Work out the finished part from the listing and answer in its coordinate system (mm). Give positions to 0.01 mm unless a question says otherwise; leave off trailing zeros. Loops run counter-clockwise (first coordinate to the right, second up) from the corner with the lowest first, then second, coordinate; pieces in that order, holes last. Notation, with made-up numbers: (58, -33.75) - (67, -33.75) arc R22 ccw to (67, -6.75) - close; hole circle Ø5 at (32, -4). An arc over 180 degrees is marked (long way). One line per question, with ' | ' between items. Start each with the question number.
1. Section A-A (z = 1.2) is taken. Give the number of separate pieces and of enclosed holes in the cut face, plus the area to 3 significant figures.
2. Section C-C (x = -40) is taken. Determine the outline of the cut face in (y, z).
3. Section B-B (y = 64.5) is taken. Determine the outline of the cut face in (x, z).
4. Find the intervals of material crossed by line 1 (X direction, y = 100, z = 1.4); line 2 (Y direction, x = 15.5, z = 1.1); line 3 (Y direction, x = 2, z = 2.5), in increasing order.
5. Each of these flat-tipped pins is pushed along its axis until it touches: pin 1 (1 mm diameter, centred on y = 129.5, z = 3, fed in from +X); pin 2 (1.2 mm diameter, centred on y = 173, z = 3, fed in from +X); pin 3 (1.2 mm diameter, centred on x = 12, z = 2.5, fed in from -Y). Where does it stop, or does it pass through?
6. For a pull along X with two mould halves and no side action, classify faces 1 (the face through (34, 195, 2)), 2 (the face through (4, 87, 0)), 3 (the face through (-1.42, 10.78, 1.97)), 4 (the face through (-65.414, -18.312, 1.972)) as released by +X, released by -X, zero draft, split by the parting line, or undercut.
from build123d import *

# Parameters (mm, degrees)
SKETCH_1_R          = 1.5
SKETCH_1_R_2        = 10.875
EXTRUDE_1_DEPTH     = 4
FILLET_3_R          = 15
FILLET_4_R          = 5
FILLET_5_R          = 1
SKETCH_2_W          = 12.5
SKETCH_2_H          = 4
SKETCH_2_R          = 1.4
EXTRUDE_2_DEPTH     = 4
FILLET_6_R          = 5
SKETCH_4_R          = 1.5
SKETCH_4_W          = 11.25
SKETCH_4_H          = 4
CUT_EXTRUDE_2_DEPTH = 227.329405955
CHAMFER_1_SIZE      = 10
FILLET_7_R          = 10
SKETCH_3_R          = 1.5
CUT_EXTRUDE_1_DEPTH = 227.329405955


with BuildPart() as part:
    # Эскиз1 → Бобышка-Вытянуть1 (new body)
    with BuildSketch(Plane.XY):
        Polygon((-100, -14.71), (-30, -22), (30, -22), (30, 171), (55, 171), (55, 176.625), (67.5, 176.625), (67.5, 183.375), (55, 183.375), (55, 189), (30, 189), (30, 203), (-30, 203), (-30, 12.58), (-100, 5.29), (-100, -3.31), (-82.5, -3.31), (-82.5, -6.11), (-100, -6.11), align=None)
        with Locations((-15.5, -15.5)):
            Circle(SKETCH_1_R, mode=Mode.SUBTRACT)
        Circle(SKETCH_1_R_2, mode=Mode.SUBTRACT)
        with Locations((15.5, -15.5)):
            Circle(SKETCH_1_R, mode=Mode.SUBTRACT)
        with Locations((-15.5, 15.5)):
            Circle(SKETCH_1_R, mode=Mode.SUBTRACT)
        with Locations((15.5, 15.5)):
            Circle(SKETCH_1_R, mode=Mode.SUBTRACT)
        with Locations((-22.25, 100)):
            Circle(SKETCH_1_R, mode=Mode.SUBTRACT)
        with Locations((2.55, 100)):
            Circle(SKETCH_1_R, mode=Mode.SUBTRACT)
    extrude(amount=EXTRUDE_1_DEPTH)

    # Скругление3
    fillet_3_edges = [part.edges().sort_by_distance(p)[0] for p in [
        (-30, 12.58, 2),
    ]]
    fillet(fillet_3_edges, radius=FILLET_3_R)

    # Скругление4
    fillet_4_edges = [part.edges().sort_by_distance(p)[0] for p in [
        (-100, -14.71, 2),
        (-100, 5.29, 2),
    ]]
    fillet(fillet_4_edges, radius=FILLET_4_R)

    # Скругление5
    fillet_5_edges = [part.edges().sort_by_distance(p)[0] for p in [
        (-100, -6.11, 2),
        (-100, -3.31, 2),
    ]]
    fillet(fillet_5_edges, radius=FILLET_5_R)

    # Эскиз2 → Бобышка-Вытянуть2 (add, through all)
    # profile 1 of 3: a face of its own
    with BuildSketch(Plane.XY.offset(4)):
        with Locations((-23.75, -24)):
            Rectangle(SKETCH_2_W, SKETCH_2_H)
        with Locations((-23.75, -23.75)):
            Circle(SKETCH_2_R, mode=Mode.SUBTRACT)
    # profile 2 of 3: a face of its own
    with BuildSketch(Plane.XY.offset(4)):
        with Locations((0, -24)):
            Rectangle(SKETCH_2_W, SKETCH_2_H)
    # profile 3 of 3: a face of its own
    with BuildSketch(Plane.XY.offset(4)):
        with Locations((23.75, -24)):
            Rectangle(SKETCH_2_W, SKETCH_2_H)
        with Locations((23.75, -23.75)):
            Circle(SKETCH_2_R, mode=Mode.SUBTRACT)
    extrude(amount=-EXTRUDE_2_DEPTH)

    # Скругление6
    # the kernel refuses this fillet: 5 mm, written as the material it adds along each edge
    with BuildSketch(Plane(origin=(-30, -22, 0), x_dir=(0, -1, 0), z_dir=(0, 0, 1))) as fillet_6_piece_1:
        with BuildLine():
            CenterArc((4.509032444, -4.974021107), FILLET_6_R, 95.843205651, 78.21128084)
            Line((-0.4640718, -4.456107822), (-0.563533885, -4.445749556))
            Line((-0.563533885, -4.445749556), (-0.099462085, 0.010358266))
            Line((-0.099462085, 0.010358266), (0, 0.1))
            ThreePointArc((0, 0.1), (2, 0.1), (3.989819351, 0.099480422))
            Line((3.989819351, 0.099480422), (4, 0))
        make_face()
    extrude(amount=4)

    # Эскиз4 → Вырез-Вытянуть2 (cut, through all)
    with BuildSketch(Plane.XY.offset(4)):
        with Locations((23.75, 180)):
            Circle(SKETCH_4_R)
        with Locations((-23.75, 180)):
            Circle(SKETCH_4_R)
        with Locations((-11.875, 180)):
            Rectangle(SKETCH_4_W, SKETCH_4_H)
        with Locations((11.875, 180)):
            Rectangle(SKETCH_4_W, SKETCH_4_H)
        with Locations((35.625, 180)):
            Rectangle(SKETCH_4_W, SKETCH_4_H)
        with Locations((47.5, 180)):
            Circle(SKETCH_4_R)
    extrude(amount=-CUT_EXTRUDE_2_DEPTH, mode=Mode.SUBTRACT)

    # Фаска1
    chamfer_1_edges = [part.edges().sort_by_distance(p)[0] for p in [
        (30, 171, 2),
        (30, 189, 2),
    ]]
    chamfer(chamfer_1_edges, length=CHAMFER_1_SIZE)

    # Скругление7
    fillet_7_edges = [part.edges().sort_by_distance(p)[0] for p in [
        (40, 171, 2),
        (40, 189, 2),
    ]]
    fillet(fillet_7_edges, radius=FILLET_7_R)

    # Эскиз3 → Вырез-Вытянуть1 (cut, through all)
    with BuildSketch(Plane.XY.offset(4)):
        with Locations((-25, 45)):
            Circle(SKETCH_3_R)
        with Locations((25, 45)):
            Circle(SKETCH_3_R)
        with Locations((-25, 35)):
            Circle(SKETCH_3_R)
        with Locations((25, 35)):
            Circle(SKETCH_3_R)
    extrude(amount=-CUT_EXTRUDE_1_DEPTH, mode=Mode.SUBTRACT)


solid = part.part
Conclusion:
1) separate pieces: 1 | enclosed holes: 19 | area: 15,600 mm²
2) outline: (-20.96, 0) - (11.96, 0) - (11.96, 4) - (-20.96, 4) - close
3) outline: (-30, 0) - (30, 0) - (30, 4) - (-30, 4) - close
4) line 1: -30 to -23.75, -20.75 to 1.05, 4.05 to 30 | line 2: -22 to -17, -14 to 14, 17 to 178, 182 to 203 | line 3: -26 to -10.69, 10.69 to 98.6, 101.4 to 203
5) pin 1: x = 30 | pin 2: x = 55 | pin 3: y = -22
6) face 1: released by +X | face 2: zero draft | face 3: undercut | face 4: released by -X
